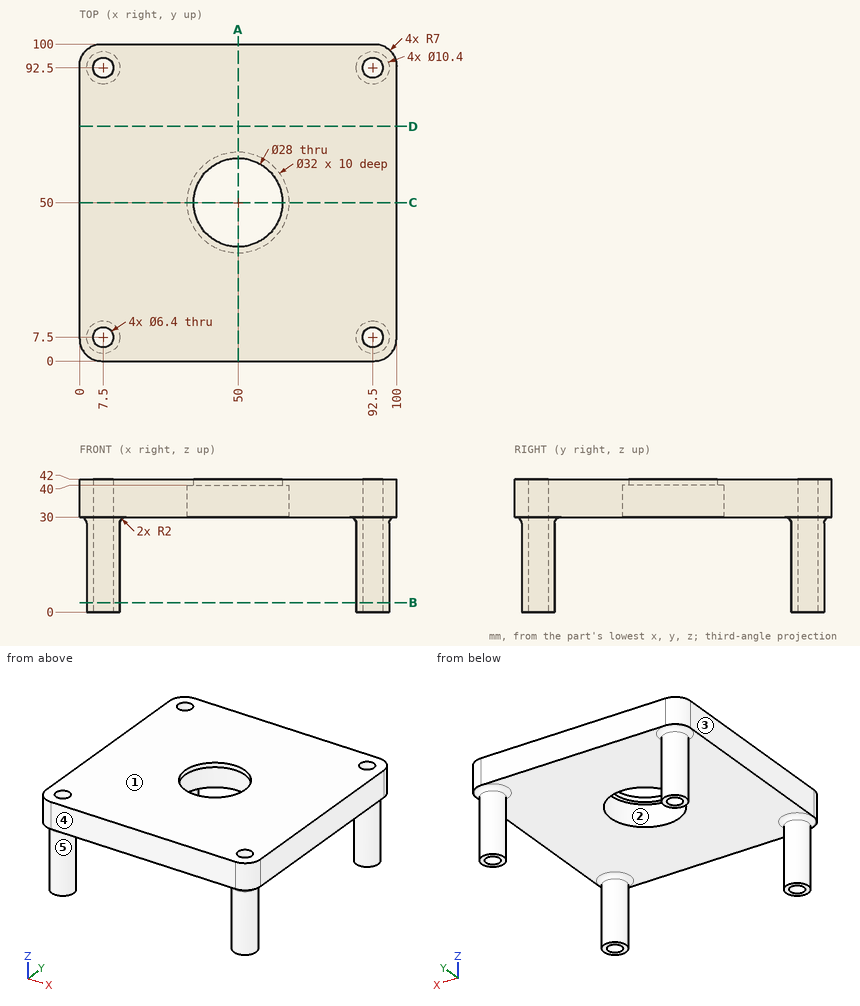
Job drawing, mm, ordinate dimensions from the low corner. One solid piece. A direction names the side the tool comes from. Coordinates: 2 decimals unless noted, no trailing zeros. Order: outer loops, then holes, each group sorted by start corner. A loop starts at its lowest first (then second) coordinate and runs counter-clockwise, first axis right, second up. Notation, with made-up numbers: (-8, 62) - (51, 62) arc R12 ccw to (51, 85) - close; hole circle Ø3 at (54, 13.5). An arc over 180 degrees is marked (long way). Write each question's results on one line, items separated by ' | '. Start each with the question number.
Item 1: Flat gauge pin, fed straight in: pin 1 (8 mm diameter, centred on x = 75.5, y = 49, fed in from -Z). Where does the tip first touch, or does it go through?
Item 2: Band-saw the part on D-D on y = 74. Write the cut outline in (x, z), and give its area (3 significant figures).
Item 3: Tool access for the marked faces 4 and 5: list every direction of +Z, -Z, +X, -X, +Y, -Y with a clear straight run to the whole face (end or side of a thin tool).
Item 4: Wall check: probe 1 along Y at (x, z) = (92.5, 35.5); probe 2 along Y at (x, z) = (50, 41.6); probe 3 along X at (y, z) = (5, 17.5). Give the ranges that are in metal, low to high. Write a range as [from, to].
Item 5: Band-saw the part on A-A on x = 50. Write the cut outline in (y, z), and give its area (3 significant figures).
Item 6: Band-saw the part on B-B on z = 3. Write the cut outline in (x, y), and give its area (3 significant figures).
Item 7: Mould opens along X. For the marked faces 1, 2 and 3 say: released by +X, released by -X, zero draft, split by the parting line, or undercut.
Numbers:
1) pin 1: z = 30
2) outline: (0, 30) - (100, 30) - (100, 42) - (0, 42) - close | area: 1,200 mm^2
3) face 4: +Z, -Z, +X, -X, -Y | face 5: -Z
4) probe 1: [0, 4.3], [10.7, 89.3], [95.7, 100] | probe 2: [0, 36], [64, 100] | probe 3: [2.94, 5.5], [9.5, 12.06], [87.94, 90.5], [94.5, 97.06]
5) outline: (0, 30) - (34, 30) - (34, 40) - (36, 40) - (36, 42) - (0, 42) - close; (64, 40) - (66, 40) - (66, 30) - (100, 30) - (100, 42) - (64, 42) - close | area: 824 mm^2
6) outline: circle Ø10.4 at (7.5, 7.5); circle Ø10.4 at (7.5, 92.5); circle Ø10.4 at (92.5, 7.5); circle Ø10.4 at (92.5, 92.5); hole circle Ø6.4 at (7.5, 7.5); hole circle Ø6.4 at (7.5, 92.5); hole circle Ø6.4 at (92.5, 7.5); hole circle Ø6.4 at (92.5, 92.5) | area: 211 mm^2
7) face 1: zero draft | face 2: undercut | face 3: released by -X
